Geometry: see drawing. Coordinates: mm, zero at the bounding-box minimum. A direction names the side the tool comes from. Give positions to 0.01 mm unless a question says otherwise; leave off trailing zeros. Order: outer loops, then holes, each group sorted by start corner. A loop starts at its lowest first (then second) coordinate and runs counter-clockwise, first axis right, second up. Notation, with made-up numbers: (67, -17) - (123, -17) arc R24 cw to (123, -7) - close; hole circle Ø9 at (82, -24). An arc over 180 degrees is marked (long way). Put each result on its own line as item: value. Start each with the question number.
1. Set-up query: the marked faces 1 and 2. Return all of +Z, -Z, +X, -X, +Y, -Y with unobstructed straight access to the full face (end or side cutting, diameter ignored); none if empty.
2. Section A-A on x = 3.75. Return the cut outline in (y, z), plus the area to 3 significant figures.
3. First-contact query: P1, Ø1, axis at y = 2.5, z = 5, coming from the +X side; P2, Ø4, axis at x = 3.5, y = 6.5, coming from the -Z side. Flat tips, straight axial feed; report the tip coordinate or a pass-through.
4. Section C-C on y = 5. Return the cut outline in (x, z).
5. Ray query, line 1 along Y through (x, z) = (0.5, 4.5); line 2 along Z through (x, y) = (5, 8.5); line 3 along X through (y, z) = (6.75, 2). Return the intervals inside material, ascending. Write a range as from..to.
6. Section B-B on z = 3.75. Return the cut outline in (x, y).
7. Section D-D on x = 1.75. Return the cut outline in (y, z), plus the area to 3 significant figures.
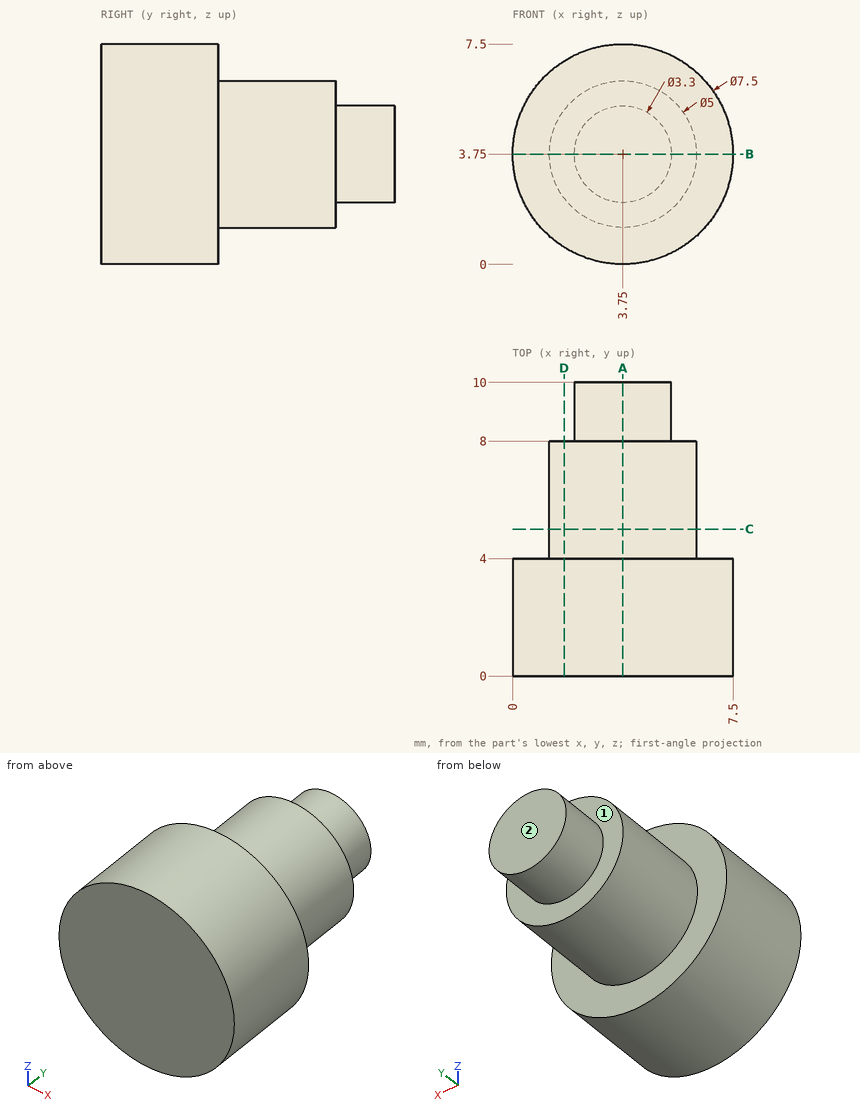
Resolved:
1. face 1: +Y
1. face 2: +Z, -Z, +X, -X, +Y
2. outline: (0, 0) - (4, 0) - (4, 1.25) - (8, 1.25) - (8, 2.1) - (10, 2.1) - (10, 5.4) - (8, 5.4) - (8, 6.25) - (4, 6.25) - (4, 7.5) - (0, 7.5) - close
2. area: 56.6 mm^2
3. P1: x = 7.42
3. P2: z = 1.25
4. outline: circle Ø5 at (3.75, 3.75)
5. line 1: 0..4
5. line 2: 2.67..4.83
5. line 3: 1.96..5.54
6. outline: (0, 0) - (7.5, 0) - (7.5, 4) - (6.25, 4) - (6.25, 8) - (5.4, 8) - (5.4, 10) - (2.1, 10) - (2.1, 8) - (1.25, 8) - (1.25, 4) - (0, 4) - close
7. outline: (0, 0.58) - (4, 0.58) - (4, 2.25) - (8, 2.25) - (8, 5.25) - (4, 5.25) - (4, 6.92) - (0, 6.92) - close
7. area: 37.4 mm^2
